```python
from build123d import *

# Parameters (mm, degrees)
SM_BASE_FLANGE_1_DEPTH = 15
CUT_EXTRUDE_1_REACH    = 31.428
SKETCH_3_R             = 2.5


# Sheet-metal steps are written as plain solids
with BuildPart() as part:
    # Sketch 1 → 基体-法兰1 (new, symmetric)
    with BuildSketch(Plane.XY):
        with BuildLine():
            Line((0, -25), (0, -1.5))
            ThreePointArc((0, -1.5), (0.439339828, -0.439339828), (1.5, 0))
            Line((1.5, 0), (5, 0))
            Line((5, 0), (5, -1))
            Line((5, -1), (1.5, -1))
            ThreePointArc((1.5, -1), (1.146446609, -1.146446609), (1, -1.5))
            Line((1, -1.5), (1, -25))
            Line((1, -25), (0, -25))
        make_face()
    extrude(amount=SM_BASE_FLANGE_1_DEPTH, both=True)

    # 草图3 → 切除-拉伸1 (cut, up to next)
    with BuildSketch(Plane(origin=(1, 0, 0), x_dir=(0, 0, -1), z_dir=(1, 0, 0)), mode=Mode.PRIVATE) as cut_extrude_1_sk1:
        with Locations((-9, -20)):
            Circle(SKETCH_3_R)
    cut_extrude_1_tool1 = extrude(cut_extrude_1_sk1.sketch, amount=-CUT_EXTRUDE_1_REACH, mode=Mode.PRIVATE) & part.part
    # 草图3 → 切除-拉伸1 (cut, up to next)
    with BuildSketch(Plane(origin=(1, 0, 0), x_dir=(0, 0, -1), z_dir=(1, 0, 0)), mode=Mode.PRIVATE) as cut_extrude_1_sk2:
        with Locations((9, -20)):
            Circle(SKETCH_3_R)
    cut_extrude_1_tool2 = extrude(cut_extrude_1_sk2.sketch, amount=-CUT_EXTRUDE_1_REACH, mode=Mode.PRIVATE) & part.part
    add(cut_extrude_1_tool1.solids().sort_by_distance((1, -20, 9))[0], mode=Mode.SUBTRACT)
    add(cut_extrude_1_tool2.solids().sort_by_distance((1, -20, -9))[0], mode=Mode.SUBTRACT)


solid = part.part
```
For this review, take the finished solid that the model builds, in its own axes (mm). A direction names the side the tool comes from. Round coordinates to 2 decimals unless told otherwise and drop trailing zeros. Write each loop counter-clockwise with the first axis right and the second up, starting at its lowest first coordinate (ties: lowest second). Pieces come first, ordered by that corner, then holes. Notation, with made-up numbers: (-13.5, -31) - (-9.5, -31) arc R20 cw to (-9.5, -1) - close; hole circle Ø4 at (-19.75, -32). An arc over 180 degrees is marked (long way). Answer as CSV lines item,"result". Start each with the question number.
(1) Add section C-C, the plane x = 3.35. State the section outline as (y, z) points.
(2) Mouldability with a two-part tool opening along Z and no side actions: class faces 3 (the cylindrical face through (0.51, -17.52, 9.33)), 4 (the flat face through (1, -13, 0)), 5 (the flat face through (0.8, -10.6, -15)), 6 (the cylindrical face through (0.51, -17.52, -8.67)) as +Z half, -Z half, draft (parallel to the pull), parting line (faces both ways), or undercut.
(3) Add section A-A, the plane z = 9. State the section outline as (x, y) points.
(4) Add section D-D, the plane z = 4.25. State the section outline as (x, y) points, plus the area to 3 significant figures.
(5) Add section B-B, the plane y = -20.75. State the section outline as (x, z) points.
(6) For pin 1 (4 mm diameter, centred on y = -11, z = -2.5, fed in from +X); pin 2 (1.8 mm diameter, centred on x = 4, z = 4, fed in from -Y), all flat-tipped, find the tip position at first contact; note any pin that passes through.
(7) Machinability: for faces 1 (the cylindrical face through (0.43, -0.45, 0.21)), 2 (the flat face through (3, -1, 0)), which of the approach directions +Z, -Z, +X, -X, +Y, -Y give a long, thin tool a straight path to every point of the face, cutting with its end or side? Answer none if there is none.
(8) For line 1 (Z direction, x = 0.55, y = -21.5); line 2 (X direction, y = -15.5, z = 6); line 3 (Y direction, x = 3.85, z = -4.75), list the stretches that pass through material, from the lowest coordinate up.
From the geometry:
1,outline,"(-1, -15) - (0, -15) - (0, 15) - (-1, 15) - close"
2,face 3,"undercut"
2,face 4,"draft"
2,face 5,"-Z half"
2,face 6,"undercut"
3,outline,"(0, -25) - (1, -25) - (1, -22.5) - (0, -22.5) - close; (0, -17.5) - (1, -17.5) - (1, -1.5) arc R0.5 cw to (1.5, -1) - (5, -1) - (5, 0) - (1.5, 0) arc R1.5 ccw to (0, -1.5) - close"
4,outline,"(0, -25) - (1, -25) - (1, -1.5) arc R0.5 cw to (1.5, -1) - (5, -1) - (5, 0) - (1.5, 0) arc R1.5 ccw to (0, -1.5) - close"
4,area,"28.6 mm²"
5,outline,"(0, -15) - (1, -15) - (1, -11.38) - (0, -11.38) - close; (0, -6.62) - (1, -6.62) - (1, 6.62) - (0, 6.62) - close; (0, 11.38) - (1, 11.38) - (1, 15) - (0, 15) - close"
6,pin 1,"stops at x = 1"
6,pin 2,"stops at y = -1"
7,face 1,"+Z, -Z, -X, +Y"
7,face 2,"+Z, -Z, +X, -Y"
8,line 1,"z = -15 to -11, -7 to 7, 11 to 15"
8,line 2,"x = 0 to 1"
8,line 3,"y = -1 to 0"
